```python
from build123d import *

# Parameters (mm, degrees)
F1_DEPTH = 38.1
F2_R     = 40.931298
F3_DEPTH = 63.5
F4_SIZE  = 5.08
F5_R     = 35.9841
F6_DEPTH = 203.2


with BuildPart() as f1:
    # F0 (on Front) → F1 (new body)
    with BuildSketch(Plane.XZ):
        Polygon((76.720704, -24.324451), (56.083392, 52.35003), (-20.637312, 72.814834), (-76.720704, 16.605157), (-56.083392, -60.069323), (20.637312, -80.534127), align=None)
    extrude(amount=F1_DEPTH)

    # F2 (on face) → F3 (join)
    with BuildSketch(Plane.XZ.offset(38.1)):
        Circle(F2_R)
    extrude(amount=F3_DEPTH)

    # F4
    f4_edges = [f1.edges().sort_by_distance(p)[0] for p in [
        (-40.931298, -101.6, 0),
    ]]
    chamfer(f4_edges, length=F4_SIZE)

    # F5 (on face) → F6 (join)
    with BuildSketch(Plane.XZ.offset(101.6)):
        Circle(F5_R)
    extrude(amount=F6_DEPTH)


solid = f1.part
```
For this review, take the finished solid that the model builds, in its own axes (mm). A direction names the side the tool comes from. Round coordinates to 2 decimals unless told otherwise and drop trailing zeros. Loops run counter-clockwise (first coordinate to the right, second up) from the corner with the lowest first, then second, coordinate; pieces in that order, holes last.
(1) We need section A-A (z = 0). Give the boundary of the cut face in (x, y), plus the area to 3 significant figures.
Returned:
outline: (-72.25, -38.1) - (-40.93, -38.1) - (-40.93, -96.52) - (-35.85, -101.6) - (-35.98, -101.6) - (-35.98, -304.8) - (35.98, -304.8) - (35.98, -101.6) - (35.85, -101.6) - (40.93, -96.52) - (40.93, -38.1) - (70.17, -38.1) - (70.17, 0) - (-72.25, 0) - close
area: 25,200 mm2
(2) We need section D-D (y = -237). Give the boundary of the cut face in (x, z), plus the area to 3 significant figures.
Returned:
outline: circle Ø71.97 at (0, 0)
area: 4,070 mm2
(3) Tool access review of faces 1 (the flat face through (-1, -304.8, 1)), 2 (the cylindrical face through (-28.556, -201.778, -21.896)): name each direction out of +Z, -Z, +X, -X, +Y, -Y from which nothing blocks a thin tool from reaching the whole face with its end or side.
Returned:
face 1: +Z, -Z, +X, -X, -Y
face 2: -Y
(4) Wall thickness on line 1 along Y through (x, z) = (-36, 27); line 2 along Z through (x, y) = (52, -31); line 3 along Z through (x, y) = (-24, -160): over which ranges is each line inside the solid? List them lowest first.
Returned:
line 1: y = -38.1 to 0
line 2: z = -49.1 to 53.44
line 3: z = -26.81 to 26.81
(5) We need section B-B (x = 0). Give the boundary of the cut face in (y, z), plus the area to 3 significant figures.
Returned:
outline: (-304.8, -35.98) - (-101.6, -35.98) - (-101.6, -35.85) - (-96.52, -40.93) - (-38.1, -40.93) - (-38.1, -75.03) - (0, -75.03) - (0, 67.31) - (-38.1, 67.31) - (-38.1, 40.93) - (-96.52, 40.93) - (-101.6, 35.85) - (-101.6, 35.98) - (-304.8, 35.98) - close
area: 25,200 mm2
(6) We need section C-C (y = -49). Give the boundary of the cut face in (x, z), plus the area to 3 significant figures.
Returned:
outline: circle Ø81.86 at (0, 0)
area: 5,260 mm2
(7) Clearance check with flat-ended pins moving along their axes: P1, Ø4, axis at x = 2.5, z = -47.5, coming from the -Y side; P2, Ø3, axis at x = -3, y = -140, coming from the -Z side; P3, Ø2, axis at y = -91, z = 27, coming from the -X side. State where each tip first meets the part, or that it passes through.
Returned:
P1: stops at y = -38.1
P2: stops at z = -35.95
P3: stops at x = -31.61
